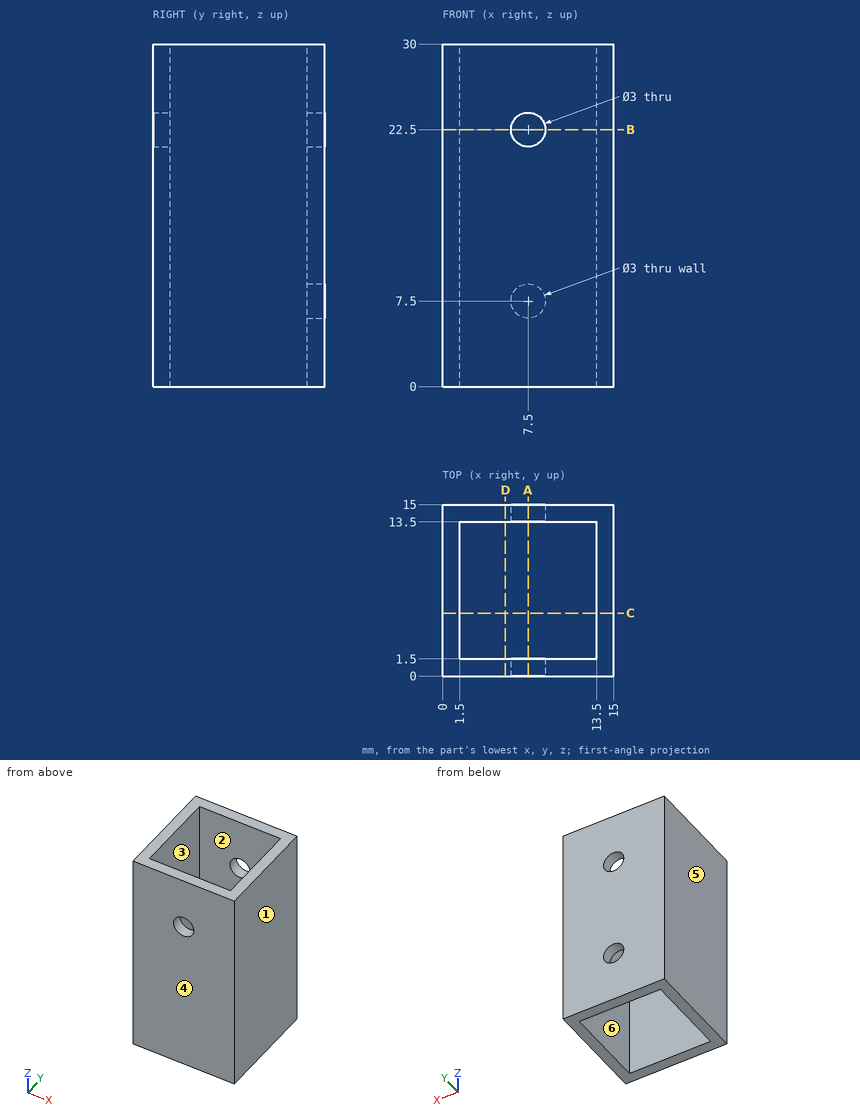
The figure shows three views and two pictorial views of one solid part (mm, origin at its lowest corner). Answer the questions. A direction names the side the tool comes from. Give positions to 0.01 mm unless a question says otherwise; leave off trailing zeros. Order: outer loops, then holes, each group sorted by start corner. A loop starts at its lowest first (then second) coordinate and runs counter-clockwise, first axis right, second up. Notation, with made-up numbers: (85, 84) - (98, 84) arc R22 cw to (98, 109) - close; hole circle Ø8 at (52.25, 75). An arc over 180 degrees is marked (long way). Answer as CSV lines item,"result".
Q1. Each of these flat-tipped pins is pushed along its axis until it touches: pin 1 Ø2.5 at (x, z) = (7.5, 22.5) entering from -Y; pin 2 Ø2.5 at (x, z) = (7.5, 7.5) entering from +Y. Where does it stop, or does it pass through?
Answer key:
pin 1,"passes through"
pin 2,"stops at y = 1.5"
Q2. A cutting plane is placed at A-A, the plane x = 7.5. Determine the outline of the cut face in (y, z), and give its area (3 significant figures).
Answer key:
outline,"(0, 0) - (1.5, 0) - (1.5, 21) - (0, 21) - close; (0, 24) - (1.5, 24) - (1.5, 30) - (0, 30) - close; (13.5, 0) - (15, 0) - (15, 6) - (13.5, 6) - close; (13.5, 9) - (15, 9) - (15, 21) - (13.5, 21) - close; (13.5, 24) - (15, 24) - (15, 30) - (13.5, 30) - close"
area,"76.5 mm^2"
Q3. Which of the six approach directions +Z, -Z, +X, -X, +Y, -Y give full straight-line access (tool end or side, diameter ignored) to the marked faces 5 and 6?
Answer key:
face 5,"+Z, -Z, -X, +Y, -Y"
face 6,"+Z, -Z"
Q4. A cutting plane is placed at B-B, the plane z = 22.5. Determine the outline of the cut face in (x, y).
Answer key:
outline,"(0, 0) - (6, 0) - (6, 1.5) - (1.5, 1.5) - (1.5, 13.5) - (6, 13.5) - (6, 15) - (0, 15) - close; (9, 0) - (15, 0) - (15, 15) - (9, 15) - (9, 13.5) - (13.5, 13.5) - (13.5, 1.5) - (9, 1.5) - close"
Q5. Straight lines are drawn through the part: L1, parallel to Z at x = 7.5, y = 14; L2, parallel to X at y = 0.7, z = 22.5; L3, parallel to X at y = 8.5, z = 21.25. For each, find the intervals that lie inside material, in ascending order.
Answer key:
L1,"z = 0 to 6, 9 to 21, 24 to 30"
L2,"x = 0 to 6, 9 to 15"
L3,"x = 0 to 1.5, 13.5 to 15"
Q6. A cutting plane is placed at C-C, the plane y = 5.5. Determine the outline of the cut face in (x, z), and give its area (3 significant figures).
Answer key:
outline,"(0, 0) - (1.5, 0) - (1.5, 30) - (0, 30) - close; (13.5, 0) - (15, 0) - (15, 30) - (13.5, 30) - close"
area,"90.0 mm^2"
Q7. Determine the mould class of the marked faces 1, 2, 3 and 4 for opening direction Y: pulls with the +Y half, pulls with the -Y half, needs draft (parallel to the pull), parting line crosses it, or undercut.
Answer key:
face 1,"needs draft"
face 2,"undercut"
face 3,"undercut"
face 4,"pulls with the -Y half"
